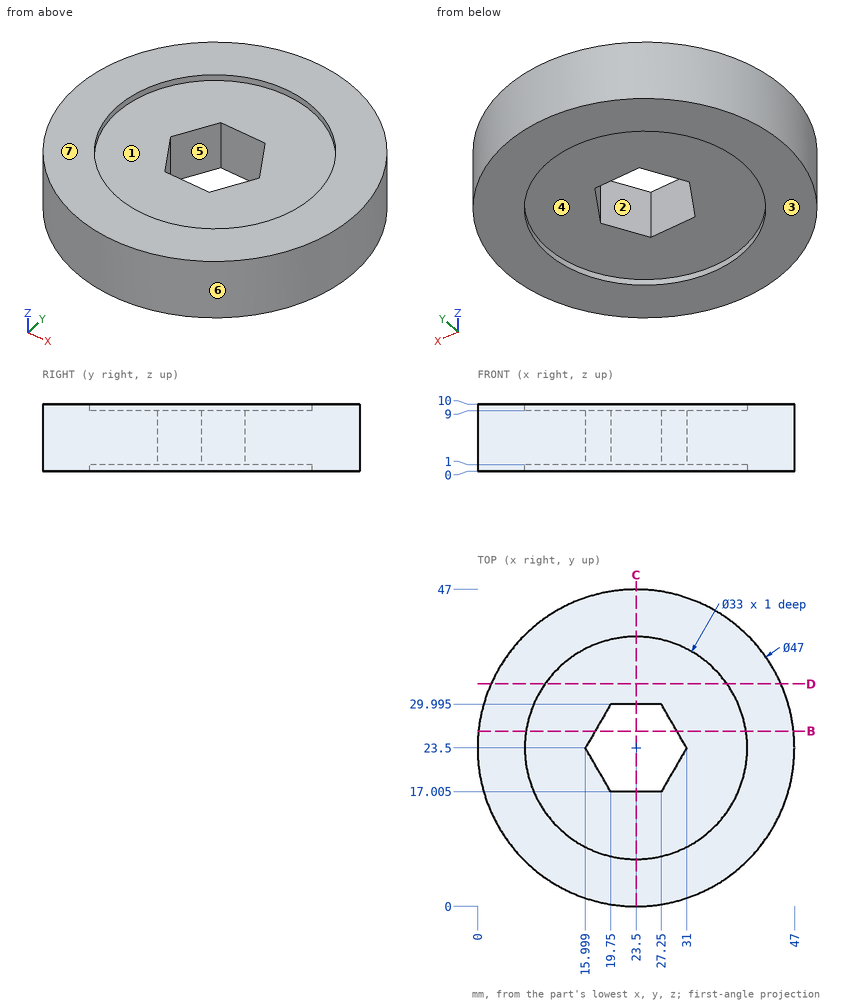
Part print with two shaded views. Sizes in mm from the minimum x, y, z corner. A direction names the side the tool comes from. Round coordinates to 2 decimals unless told otherwise and drop trailing zeros. Loops run counter-clockwise (first coordinate to the right, second up) from the corner with the lowest first, then second, coordinate; pieces in that order, holes last. Notation, with made-up numbers: M 48,0 L 58,0 A27 ccw 58,18 Z; hole C 60,73.25 d3. An arc over 180 degrees is marked long. Return JSON: item names as keys, results as strings. Group by question number.
(1) Saw through at C-C, the plane x = 23.5. List the corners of the cut face in (y, z) (1 decimal).
(2) Wall check: probe 1 along Y at (x, z) = (23.5, 0.55); probe 2 along Z at (x, y) = (30, 17.5); probe 3 along X at (y, z) = (29, 3.5) (1 decimal). Give the ranges that are in metal, low to high. Write a range as [from, to].
(3) Tool access for the marked faces 1, 2, 3 and 4: list every direction of +Z, -Z, +X, -X, +Y, -Y with a clear straight run to the whole face (end or side of a thin tool).
(4) Saw through at B-B, the plane y = 26. List the corners of the cut face in (x, z).
(5) Saw through at D-D, the plane y = 33. List the corners of the cut face in (x, z), and give its area (3 significant figures).
(6) Mould opens along X. For the marked faces 5, 6 and 7 say: +X half, -X half, draft (parallel to the pull), parting line (faces both ways), or undercut.
(7) Drop flat-ended pins along their axis: P1, Ø4, axis at y = 25.5, z = 2.5, coming from the -X side; P2, Ø2, axis at x = 24.5, z = 5.5, coming from the +Y side; P3, Ø4, axis at x = 17, z = 7, coming from the +Y side (1 decimal); P4, Ø3, axis at y = 10, z = 8, coming from the -X side (1 decimal). Give the stop position or say it passes through.
Answer list:
{
 "1": {"outline": "M 0,0 L 7,0 L 7,1 L 17,1 L 17,9 L 7,9 L 7,10 L 0,10 Z; M 30,1 L 40,1 L 40,0 L 47,0 L 47,10 L 40,10 L 40,9 L 30,9 Z"},
 "2": {"probe 1": "[0, 7], [40, 47]", "probe 2": "[1, 9]", "probe 3": "[0.7, 19.2], [27.8, 46.3]"},
 "3": {"face 1": "+Z", "face 2": "+Z, -Z", "face 3": "-Z, +X, -X, +Y, -Y", "face 4": "-Z"},
 "4": {"outline": "M 0.13,0 L 7.19,0 L 7.19,1 L 17.44,1 L 17.44,9 L 7.19,9 L 7.19,10 L 0.13,10 Z; M 29.56,1 L 39.81,1 L 39.81,0 L 46.87,0 L 46.87,10 L 39.81,10 L 39.81,9 L 29.56,9 Z"},
 "5": {"outline": "M 2.01,0 L 10.01,0 L 10.01,1 L 36.99,1 L 36.99,0 L 44.99,0 L 44.99,10 L 36.99,10 L 36.99,9 L 10.01,9 L 10.01,10 L 2.01,10 Z", "area": "376 mm2"},
 "6": {"face 5": "undercut", "face 6": "parting line", "face 7": "draft"},
 "7": {"P1": "x = 0", "P2": "y = 47", "P3": "y = 46.6", "P4": "x = 3.3"}
}
